Here's how the part is built. I have some questions about the finished solid (model axes, mm). Round coordinates to 2 decimals unless told otherwise and drop trailing zeros. Order: outer loops, then holes, each group sorted by start corner. A loop starts at its lowest first (then second) coordinate and runs counter-clockwise, first axis right, second up. Notation, with made-up numbers: (50, 36.25) -> (93, 36.25) arc R28 ccw to (93, 62.25) -> close; hole circle Ø8 at (68, 8.5). An arc over 180 degrees is marked (long way). One line per item, written item: value.
```python
from build123d import *

# Parameters (mm, degrees)
F1_DEPTH = 4
F2_W     = 93
F2_H     = 45
F3_DEPTH = 25


with BuildPart() as f1:
    # F0 (on Top) → F1 (new body)
    with BuildSketch(Plane.XY):
        with BuildLine():
            Line((-543.323108, 495), (543.323108, 495))
            ThreePointArc((543.323108, 495), (0, 735), (-543.323108, 495))
        make_face()
    extrude(amount=F1_DEPTH)

    # F2 (on face) → F3 (cut)
    with BuildSketch(Plane.XY.offset(4)):
        with Locations((196.5, 517.5)):
            Rectangle(F2_W, F2_H)
        with Locations((-196.5, 517.5)):
            Rectangle(F2_W, F2_H)
    extrude(amount=-F3_DEPTH, mode=Mode.SUBTRACT)


solid = f1.part
```
Q1. I want a section at A-A on z = 2.85. Write out the boundary of the cut face in (x, y).
Answers:
outline: (-543.32, 495) -> (-243, 495) -> (-243, 540) -> (-150, 540) -> (-150, 495) -> (150, 495) -> (150, 540) -> (243, 540) -> (243, 495) -> (543.32, 495) arc R735 ccw to start
Q2. I want a section at B-B on y = 513.5. Write out the boundary of the cut face in (x, z), then the cut area to 3 significant figures.
Answers:
outline: (-525.87, 0) -> (-243, 0) -> (-243, 4) -> (-525.87, 4) -> close; (-150, 0) -> (150, 0) -> (150, 4) -> (-150, 4) -> close; (243, 0) -> (525.87, 0) -> (525.87, 4) -> (243, 4) -> close
area: 3,460 mm2
Q3. For P1, Ø1, axis at y = 530, z = 2, coming from the -X side; P2, Ø2, axis at y = 514, z = 2, coming from the -X side; P3, Ø2, axis at x = -198.5, z = 1.5, coming from the -Y side, each with a flat end and sliding along its axis, tell me the tip position at first contact or that it passes through.
Answers:
P1: x = -509.76
P2: x = -526.36
P3: y = 540
Q4. I want a section at C-C on x = -413. Write out the boundary of the cut face in (y, z).
Answers:
outline: (495, 0) -> (607.99, 0) -> (607.99, 4) -> (495, 4) -> close
Q5. I need wall thicknesses on line 1 along Y through (x, z) = (-362.5, 0.45); line 2 along X through (y, z) = (545, 2.8); line 3 along X through (y, z) = (563, 1.2). Which ranges of each line are inside material? Lowest first, please.
Answers:
line 1: 495 to 639.39
line 2: -493.15 to 493.15
line 3: -472.5 to 472.5
Q6. I want a section at D-D on y = 619.5. Write out the boundary of the cut face in (x, z), then the cut area to 3 significant figures.
Answers:
outline: (-395.53, 0) -> (395.53, 0) -> (395.53, 4) -> (-395.53, 4) -> close
area: 3,160 mm2
